Source: CAD feature listing. Evaluate the final solid. Frame: model axes, mm. Round coordinates to 2 decimals unless told otherwise and drop trailing zeros. Order: outer loops, then holes, each group sorted by start corner. A loop starts at its lowest first (then second) coordinate and runs counter-clockwise, first axis right, second up. Notation, with made-up numbers: (15, 84) -> (48, 84) arc R30 ccw to (48, 109) -> close; hole circle Ø6 at (62, 38). An arc over 180 degrees is marked (long way). One line per item, written item: value. Start each with the question number.
1) Section B-B (y = 0.8). State how many separate pieces and enclosed holes the cut face has, and give its area (3 significant figures).
2) Section C-C (z = -36). Return the cut outline in (x, y), and give its area (3 significant figures).
3) Ray query, L1, parallel to X at y = 1.95, z = 4; L2, parallel to Z at x = -5, y = 1.85; L3, parallel to X at y = 1.75, z = 13. Return the intervals inside material, ascending.
4) Section A-A (x = -31). Return the cut outline in (y, z), and give its area (3 significant figures).
5) Mould query, pull axis Z, two halves, no side actions, for faces 1 (the face through (9.297, 1.521, -128.986)), 2 (the face through (-29.5, 1.5, -129.2)), 3 (the face through (-73.09, 1.48, -114.01)), 4 (the face through (-89.297, 1.521, 26.986)). Classes: pulls with the +Z half, pulls with the -Z half, needs draft (parallel to the pull), parting line crosses it, or undercut.
6) Section D-D (x = 7). Return the cut outline in (y, z).
Autodesk Inventor part; units mm, degrees
ref_plane "Work Plane1" through (-75, 0, -51) normal (0, 0, 1) x (1, 0, 0)
ref_plane "Work Plane2" through (-40, 0, 13) normal (1, 0, 0) x (0, 0, -1)
ref_plane "Work Plane3" through (7, 3, -104.15) normal (1, 0, 0) x (0, 0, -1)
sketch "Sketch1" plane through (0, 0, 0) normal (0, 1, 0) x (-1, 0, 0)
  line L0 (-15, 33) -> (95, 33)
  line L1 (95, 33) -> (95, -135)
  line L2 (95, -135) -> (-15, -135)
  line L3 (-15, -135) -> (-15, 33)
  line L4 (95, 33) -> (95, 15)
  line L5 (-15, 33) -> (-15, 13)
  line L6 (95, -135) -> (95, -115)
  line L7 (-15, -135) -> (-15, -115)
  line L8 (40, -135) -> (40, -130)
  line L9 (31, -130) -> (49, -130)
  line L10 (49, -130) -> (49, -106)
  line L11 (49, -106) -> (31, -106)
  line L12 (31, -106) -> (31, -130)
  line L13 (40, 33) -> (40, 28)
  line L14 (31, 28) -> (49, 28)
  line L15 (49, 28) -> (49, 4)
  line L16 (49, 4) -> (31, 4)
  line L17 (31, 4) -> (31, 28)
  point P0 (0, 0)
  point P1 (47.5, 33)
  point P2 (12.5, 33)
  point P3 (67.5, -135)
  point P4 (32.5, -135)
  dimension "d21" = 0
  dimension "d4" = 110
  dimension "d5" = 168
  dimension "d22" = 5
  dimension "d23" = 18
  dimension "d24" = 24
  dimension "d25" = 5
  dimension "d26" = 18
  dimension "d27" = 24
extrude "Extrusion2" add sketch "Sketch1" along normal blind 3 contours L9 L12 L11 L10 | L14 L15 L16 L17 | L0 L1 L2 L3
hole "Hole1" at (-49, 0, 28) at (-49, 0, 4) at (-31, 0, 28) at (-31, 0, 4) at (-49, 0, -130) at (-31, 0, -130) at (-31, 0, -106) at (-49, 0, -106) direction (0, -1, 0) diameter 3.4 end through all both
fillet "Fillet1" radius 20 4 edges at (15, 1.5, 33) (-95, 1.5, 33) (15, 1.5, -135) (-95, 1.5, -135)
ref_plane "Work Plane1" through (-75, 0, -51) normal (0, 0, 1) x (1, 0, 0)
ref_plane "Work Plane2" through (-40, 0, 13) normal (1, 0, 0) x (0, 0, -1)
sketch "Sketch2" plane through (0, 3, 0) normal (0, 1, 0) x (1, 0, 0)
  arc A0 (-95, -13) -> (-75, -33) centre (-75, -13) ccw
  line L0 (-95, -33) -> (-95, -13)
  line L1 (-75, -33) -> (-5, -33)
  line L2 (-95, -33) -> (-75, -33)
  line L3 (-75, -33) -> (-75, -13)
  line L4 (-75, -13) -> (-95, -13)
  arc A1 (-5, -33) -> (15, -13) centre (-5, -13) ccw
  line L5 (15, -33) -> (-5, -33)
  line L6 (15, -33) -> (15, -13)
  line L7 (-5, -33) -> (-5, -13)
  line L8 (-5, -13) -> (15, -13)
  arc A2 (15, 115) -> (-5, 135) centre (-5, 115) ccw
  line L9 (15, 135) -> (15, 115)
  line L10 (15, 135) -> (-5, 135)
  line L11 (-5, 135) -> (-5, 115)
  line L12 (-5, 115) -> (15, 115)
  arc A3 (-75, 135) -> (-95, 115) centre (-75, 115) ccw
  line L13 (-95, 135) -> (-95, 115)
  line L14 (-95, 135) -> (-75, 135)
  line L15 (-95, 115) -> (-95, -13)
  line L16 (-95, 115) -> (-75, 115)
  line L17 (-75, 115) -> (-75, 135)
  point P0 (0, 0)
hole "Hole2" at (-75, 3, 13) at (-75, 3, -115) at (-5, 3, -115) at (-5, 3, 13) direction (0, -1, 0) diameter 4.3 end through all
sketch "Sketch4" plane through (0, 3, 0) normal (0, 1, 0) x (1, 0, 0)
  line L0 (15, -13) -> (15, 115)
  line L1 (15, 0) -> (7, 0)
  line L2 (-95, 115) -> (-95, -13)
  line L3 (15, 0) -> (15, 102)
  line L4 (15, 102) -> (7, 102)
  line L5 (7, 0) -> (7, 102)
  line L6 (7, 0) -> (7, 102) construction
  line L7 (9.15, 0) -> (9.15, 102)
  line L8 (4.85, 102) -> (4.85, 0)
  arc A0 (4.85, 0) -> (9.15, 0) centre (7, 0) ccw
  arc A1 (9.15, 102) -> (4.85, 102) centre (7, 102) ccw
  point P0 (0, 0)
  point P1 (7, 51)
  dimension "d45" = 8
  dimension "d46" = 102
  dimension "d47" = 8
  dimension "d48" = 4.3
extrude "Extrusion3" cut sketch "Sketch4" against normal through all contours A0 L8 A1 L4 L5 L1 | L1 L5 L4 L7
ref_plane "Work Plane3" through (7, 3, -104.15) normal (1, 0, 0) x (0, 0, -1)
properties part number "BedHousingFrame"
Findings:
1. separate pieces: 1
1. enclosed holes: 13
1. area: 17,600 mm2
2. outline: (-95, 0) -> (4.85, 0) -> (4.85, 3) -> (-95, 3) -> close; (9.15, 0) -> (15, 0) -> (15, 3) -> (9.15, 3) -> close
2. area: 317 mm2
3. L1: -95 to -50.7, -47.3 to -32.7, -29.3 to 15
3. L2: -135 to -117.15, -112.85 to 10.85, 15.15 to 33
3. L3: -95 to -77.15, -72.85 to -7.15, -2.85 to 15
4. outline: (0, -135) -> (3, -135) -> (3, -131.7) -> (0, -131.7) -> close; (0, -128.3) -> (3, -128.3) -> (3, -107.7) -> (0, -107.7) -> close; (0, -104.3) -> (3, -104.3) -> (3, 2.3) -> (0, 2.3) -> close; (0, 5.7) -> (3, 5.7) -> (3, 26.3) -> (0, 26.3) -> close; (0, 29.7) -> (3, 29.7) -> (3, 33) -> (0, 33) -> close
4. area: 463 mm2
5. face 1: pulls with the -Z half
5. face 2: undercut
5. face 3: undercut
5. face 4: pulls with the +Z half
6. outline: (0, -131) -> (3, -131) -> (3, -104.15) -> (0, -104.15) -> close; (0, 2.15) -> (3, 2.15) -> (3, 29) -> (0, 29) -> close
